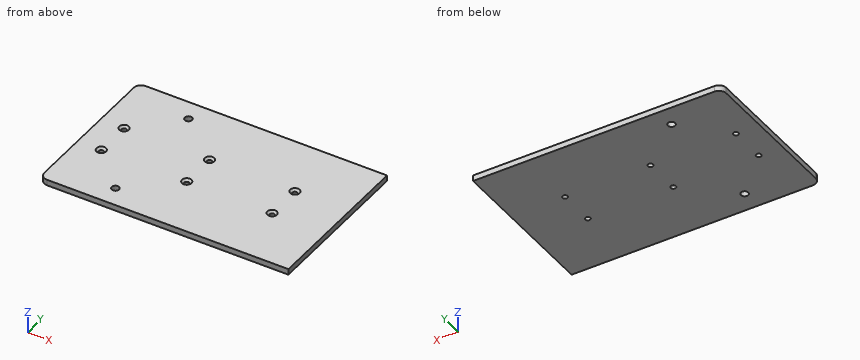
```python
from build123d import *

# Parameters (mm, degrees)
F0_W           = 170
F0_H           = 54
F1_DEPTH       = 4
F3_D           = 5
F4_D           = 3.5
F4_CSINK_D     = 6.5
F4_CSINK_ANGLE = 90
F6_R           = 5


with BuildPart() as f1:
    # F0 (on Top) → F1 (new body)
    with BuildSketch(Plane.XY):
        with Locations((10.4193558595, 27)):
            Rectangle(F0_W, F0_H)
    extrude(amount=F1_DEPTH)

    # F3 (through all)
    with Locations(Plane.XY.offset(4)):
        with Locations((-31.5806441405, 40)):
            Hole(F3_D / 2)

    # F4 (through all)
    with Locations(Plane.XY.offset(4)):
        with Locations((-58.4, 12.5), (0, 12.5), (58.4, 12.5)):
            CounterSinkHole(F4_D / 2, F4_CSINK_D / 2, counter_sink_angle=F4_CSINK_ANGLE)

    # F5: F1 across face


with BuildPart() as f1_1:
    add(f1.part)
    add(f1.part.mirror(Plane(origin=(10.4193558595, 0, 2), x_dir=(1, 0, 0), z_dir=(0, -1, 0))))

    # F6
    f6_edges = [f1_1.edges().sort_by_distance(p)[0] for p in [
        (-74.580644, 54, 2),
        (-74.580644, -54, 2),
    ]]
    fillet(f6_edges, radius=F6_R)


solid = f1_1.part
```
CAD build for the part. Positions are in the model's coordinates, mm. Round coordinates to 2 decimals unless told otherwise and drop trailing zeros. Write each loop counter-clockwise with the first axis right and the second up, starting at its lowest first coordinate (ties: lowest second). Pieces come first, ordered by that corner, then holes. Notation, with made-up numbers: (-17.75, 58.5) -> (30.25, 58.5) arc R15 ccw to (30.25, 83.5) -> close; hole circle Ø6 at (54.5, 30.25). An arc over 180 degrees is marked (long way). Answer in a Markdown table with one row per item. Add a question column.
Item 1: Saw through at C-C, the plane y = -40. Write the cut outline in (x, z).
Item 2: Saw through at B-B, the plane x = 58.4. Write the cut outline in (y, z), then the cut area to 4 significant figures.
Item 3: Drill centre lines: line 1 (Y direction, x = -58.4, z = 0.7); line 2 (X direction, y = 12.5, z = 0.6); line 3 (X direction, y = -13, z = 3.1). Where is each one in solid material? Low to high. Write a range as from..to.
Item 4: Drop a flat-ended pin along its axis: pin 1 Ø4 at (x, y) = (-58.4, -12.5) entering from +Z. Give the stop position or say it passes through.
Item 5: Saw through at A-A, the plane y = 12.5. Write the cut outline in (x, z), then the cut area to 3 significant figures.
Findings below:
| question | item | result |
|---|---|---|
| 1 | outline | (-74.58, 0) -> (-34.08, 0) -> (-34.08, 4) -> (-74.58, 4) -> close; (-29.08, 0) -> (95.42, 0) -> (95.42, 4) -> (-29.08, 4) -> close |
| 2 | outline | (-54, 0) -> (-14.25, 0) -> (-14.25, 2.5) -> (-15.75, 4) -> (-54, 4) -> close; (-10.75, 0) -> (10.75, 0) -> (10.75, 2.5) -> (9.25, 4) -> (-9.25, 4) -> (-10.75, 2.5) -> close; (14.25, 0) -> (54, 0) -> (54, 4) -> (15.75, 4) -> (14.25, 2.5) -> close |
| 2 | area | 399.5 mm^2 |
| 3 | line 1 | y = -54..-14.25, -10.75..10.75, 14.25..54 |
| 3 | line 2 | x = -74.58..-60.15, -56.65..-1.75, 1.75..56.65, 60.15..95.42 |
| 3 | line 3 | x = -74.58..-60.7, -56.1..-2.3, 2.3..56.1, 60.7..95.42 |
| 4 | pin 1 | stops at z = 2.75 |
| 5 | outline | (-74.58, 0) -> (-60.15, 0) -> (-60.15, 2.5) -> (-61.65, 4) -> (-74.58, 4) -> close; (-56.65, 0) -> (-1.75, 0) -> (-1.75, 2.5) -> (-3.25, 4) -> (-55.15, 4) -> (-56.65, 2.5) -> close; (1.75, 0) -> (56.65, 0) -> (56.65, 2.5) -> (55.15, 4) -> (3.25, 4) -> (1.75, 2.5) -> close; (60.15, 0) -> (95.42, 0) -> (95.42, 4) -> (61.65, 4) -> (60.15, 2.5) -> close |
| 5 | area | 631 mm^2 |
